Input: part model. Units: mm. Frame: model coordinates. Coordinates: 2 decimals unless noted, no trailing zeros. Loops run counter-clockwise (first coordinate to the right, second up) from the corner with the lowest first, then second, coordinate; pieces in that order, holes last. Notation, with made-up numbers: (19.25, 56) -> (34.25, 56) arc R37 cw to (34.25, 92) -> close; hole circle Ø5 at (74, -35). An arc over 180 degrees is marked (long way). Put each result on its own line as item: value. Start each with the question number.
1) Pull-direction query (X, two-part tool) for faces 1 (the flat face through (-25.4, 0, 0)), 2 (the conical face through (-11.653, 5.438, -1.712)), 3 (the cylindrical face through (-3.855, -0.991, -7.545)), 4 (the flat face through (0, 0, 0)); classes: pulls with the +X half, pulls with the -X half, needs draft (parallel to the pull), parting line crosses it, or undercut.
2) Contact query for flat-ended pins moving along their axis: P1, Ø1.5, axis at x = -17.5, y = 1, coming from the +Z side; P2, Ø5, axis at x = -21, z = 2, coming from the -Y side; P3, Ø8, axis at x = -17.5, y = 6, coming from the +Z side. Output: stop coordinate, or through.
3) Cut plane C-C (x = -4). Return the cut outline in (y, z), plus the area to 3 significant figures.
4) Material intervals for L1, parallel to Y at x = -18, z = -1.75; L2, parallel to Y at x = -14, z = -1; L3, parallel to X at y = -4, z = -1.5, sorted ascending.
5) Cut plane D-D (x = -23.5). Return the cut outline in (y, z), plus the area to 3 significant figures.
from build123d import *


with BuildPart() as f1:
    # F0 (on Top) → F1 (revolve)
    with BuildSketch(Plane.XY):
        with BuildLine():
            Line((-25.4, 0), (0, 0))
            Line((0, 0), (0, 3.006029))
            ThreePointArc((0, 3.006029), (-0.021354, 3.169318), (-0.083979, 3.321625))
            Line((-0.083979, 3.321625), (-2.357062, 7.290364))
            ThreePointArc((-2.357062, 7.290364), (-2.589633, 7.524145), (-2.908083, 7.609769))
            Line((-2.908083, 7.609769), (-4.775419, 7.609769))
            ThreePointArc((-4.775419, 7.609769), (-5.050043, 7.547313), (-5.270645, 7.37223))
            Line((-5.270645, 7.37223), (-6.536468, 5.795051))
            ThreePointArc((-6.536468, 5.795051), (-7.77584, 4.955551), (-9.272766, 4.959825))
            Line((-9.272766, 4.959825), (-17.629906, 7.563013))
            ThreePointArc((-17.629906, 7.563013), (-17.779944, 7.590558), (-17.932223, 7.581525))
            ThreePointArc((-17.932223, 7.581525), (-21.296409, 7.256235), (-24.667976, 7.493079))
            ThreePointArc((-24.667976, 7.493079), (-25.178288, 7.347632), (-25.4, 6.865535))
            Line((-25.4, 6.865535), (-25.4, 0))
        make_face()
    revolve(axis=Axis((-12.7, 0, 0), (-1, 0, 0)))


solid = f1.part
Results found:
1. face 1: pulls with the -X half
1. face 2: undercut
1. face 3: needs draft
1. face 4: pulls with the +X half
2. P1: stops at z = 7.59
2. P2: stops at y = -7.4
2. P3: stops at z = 7.32
3. outline: circle Ø15.22 at (0, 0)
3. area: 182 mm2
4. L1: y = -7.36 to 7.36
4. L2: y = -6.35 to 6.35
4. L3: x = -25.4 to -0.63
5. outline: circle Ø14.69 at (0, 0)
5. area: 170 mm2
